Part model, mm, in its own coordinate system. A direction names the side the tool comes from. Give positions to 0.01 mm unless a question says otherwise; leave off trailing zeros. Write each loop counter-clockwise with the first axis right and the second up, starting at its lowest first coordinate (ties: lowest second). Pieces come first, ordered by that corner, then holes. Notation, with made-up numbers: M -28,37 L -4,37 A6 cw -4,42 Z; hole C 53.5,56.5 d3. An arc over 180 degrees is marked long. Use CSV: the item, a comma, the result in double quotes. Start each with the question number.
Item 1: Which spindle directions (+Z, -Z, +X, -X, +Y, -Y) get a long thin tool onto all of the face, cutting with end or side? Do faces 1 (the flat face through (28, -18.336, 8)), 2 (the flat face through (22.3, -14, 8)), 3 (the cylindrical face through (35.826, -13.102, 7.569)). Say none if no direction does.
Item 2: Pin check, flat tips, straight feed: pin 1 (5 mm diameter, centred on x = 29, z = 6, fed in from +Y); pin 2 (5 mm diameter, centred on x = 19, z = 5, fed in from -Y); pin 3 (3.5 mm diameter, centred on y = -3, z = 6, fed in from -X). Stop position of each tip, or through.
Item 3: Drill centre lines: line 1 (Y direction, x = 21.5, z = 13); line 2 (X direction, y = -9, z = 13); line 3 (Y direction, x = 8.7, z = 0.65). Where is each one in solid material? Low to high. Write a range as [from, to].
Item 4: Cut at D-D (y = -9.5). List the corners of the cut face in (x, z).
Item 5: Cut at A-A (y = -2.3). List the corners of the cut face in (x, z), then the cut area to 3 significant figures.
Item 6: Cut at C-C (x = 5). List the corners of the cut face in (y, z), then the cut area to 3 significant figures.
Item 7: Mould opens along Y. For faces 4 (the flat face through (33.5, -14, 8)), 5 (the flat face through (16, -7.536, 8)), 6 (the cylindrical face through (38.8, -18.2, 0.6)), 7 (the flat face through (17, -1.036, 8)) say: released by +Y, released by -Y, zero draft, split by the parting line, or undercut.
Item 8: Cut at B-B (z = 9.75). List the corners of the cut face in (x, y).
from build123d import *

# Parameters (mm, degrees)
F0_W     = 43.688
F0_H     = 21.336
F1_DEPTH = 1.16
F2_R     = 1.7
F3_DEPTH = 25
F4_R     = 4
F4_W     = 12.3
F4_H     = 12.3
F4_W_2   = 10
F4_H_2   = 8.3
F4_W_3   = 9.5
F4_H_3   = 4.5
F5_DEPTH = 13


with BuildPart() as f1:
    # F0 (on Top) → F1 (new body)
    with BuildSketch(Plane.XY):
        with Locations((21.844, -10.668)):
            Rectangle(F0_W, F0_H)
    extrude(amount=F1_DEPTH)

    # F2 (on face) → F3 (cut)
    with BuildSketch(Plane.XY.offset(1.16)):
        with Locations((37.188, -18.736)):
            Circle(F2_R)
        with Locations((8.7, -2.3)):
            Circle(F2_R)
    extrude(amount=-F3_DEPTH, mode=Mode.SUBTRACT)

    # F4 (on face) → F5 (join)
    with BuildSketch(Plane.XY.offset(1.16)):
        with Locations((5, -10.668)):
            Circle(F4_R)
        with Locations((39, -10.668)):
            Circle(F4_R)
        with Locations((16.15, -13.686)):
            Rectangle(F4_W, F4_H)
        with Locations((28.5, -14.186)):
            Rectangle(F4_W_2, F4_H_2)
        with Locations((17.25, -3.286)):
            Rectangle(F4_W_3, F4_H_3)
    extrude(amount=F5_DEPTH)


solid = f1.part
Worked answers:
1,face 1,"+Z, +X, -Y"
1,face 2,"+Z, +Y, -Y"
1,face 3,"+Z"
2,pin 1,"stops at y = -10.04"
2,pin 2,"stops at y = -19.84"
2,pin 3,"stops at x = 12.5"
3,line 1,"y = [-19.84, -7.54], [-5.54, -1.04]"
3,line 2,"x = [1.36, 8.64], [10, 22.3], [35.36, 42.64]"
3,line 3,"y = [-21.34, -4], [-0.6, 0]"
4,outline,"M 0,0 L 43.69,0 L 43.69,1.16 L 42.83,1.16 L 42.83,14.16 L 35.17,14.16 L 35.17,1.16 L 22.3,1.16 L 22.3,14.16 L 10,14.16 L 10,1.16 L 8.83,1.16 L 8.83,14.16 L 1.17,14.16 L 1.17,1.16 L 0,1.16 Z"
5,outline,"M 0,0 L 7,0 L 7,1.16 L 0,1.16 Z; M 10.4,0 L 43.69,0 L 43.69,1.16 L 22,1.16 L 22,14.16 L 12.5,14.16 L 12.5,1.16 L 10.4,1.16 Z"
5,area,"170 mm^2"
6,outline,"M -21.34,0 L 0,0 L 0,1.16 L -6.67,1.16 L -6.67,14.16 L -14.67,14.16 L -14.67,1.16 L -21.34,1.16 Z"
6,area,"129 mm^2"
7,face 4,"zero draft"
7,face 5,"undercut"
7,face 6,"undercut"
7,face 7,"released by +Y"
8,outline,"C 5,-10.67 d8; M 10,-19.84 L 22.3,-19.84 L 22.3,-7.54 L 10,-7.54 Z; M 12.5,-5.54 L 22,-5.54 L 22,-1.04 L 12.5,-1.04 Z; M 23.5,-18.34 L 33.5,-18.34 L 33.5,-10.04 L 23.5,-10.04 Z; C 39,-10.67 d8"
